Could you check a few things on this model? Use its own coordinates, in mm. A direction names the side the tool comes from. Coordinates: 2 decimals unless noted, no trailing zeros. Write each loop counter-clockwise with the first axis right and the second up, starting at its lowest first coordinate (ties: lowest second). Pieces come first, ordered by that corner, then holes. Notation, with made-up numbers: (0.25, -24.75) - (32.25, -24.75) arc R11 cw to (32.25, -5.75) - close; hole circle Ø1 at (74.25, -17). An arc over 180 degrees is marked (long way). Write item = value, one per line. Start each with the question number.
```python
from build123d import *

# Parameters (mm, degrees)
BOSS_EXTRUDE1_DEPTH = 10
SKETCH2_R           = 7.5
BOSS_EXTRUDE2_DEPTH = 126
CHAMFER1_SIZE       = 1


with BuildPart() as part:
    # Sketch1 → Boss-Extrude1 (new body)
    with BuildSketch(Plane(origin=(0, 0, 0), x_dir=(1, 0, 0), z_dir=(0, 1, 0))):
        Polygon((0, 12.701705922), (-11, 6.350852961), (-11, -6.350852961), (0, -12.701705922), (11, -6.350852961), (11, 6.350852961), align=None)
    extrude(amount=BOSS_EXTRUDE1_DEPTH)

    # Sketch2 → Boss-Extrude2 (add)
    with BuildSketch(Plane.XZ):
        Circle(SKETCH2_R)
    extrude(amount=BOSS_EXTRUDE2_DEPTH)

    # Sketch4 → Cut-Revolve2 (revolve, cut)
    with BuildSketch(Plane(origin=(0, 0, 0), x_dir=(0, 0, -1), z_dir=(1, 0, 0))):
        Polygon((-12.701705922, 10), (-12.701705922, 8.8), (-11.201705922, 10), align=None)
        Polygon((-12.701705922, 0), (-12.701705922, 1.2), (-11.201705922, 0), align=None)
    revolve(axis=Axis((0, 0, 0), (0, 1, 0)), mode=Mode.SUBTRACT)

    # Chamfer1
    chamfer1_edges = [part.edges().sort_by_distance(p)[0] for p in [
        (-7.5, -126, 0),
    ]]
    chamfer(chamfer1_edges, length=CHAMFER1_SIZE)


solid = part.part
```
1) If I drill on probe 1 along Y at (x, z) = (4.5, 6.75); probe 2 along Z at (x, y) = (0.25, -118); probe 3 along Z at (x, y) = (-6.25, -40.5), over which ranges is the centre line in solid material (lowest first)? Write a range as [from, to].
2) For P1, Ø3, axis at x = 7, y = -19, coming from the -Z side; P2, Ø10, axis at x = -6, y = -28, coming from the -Z side; P3, Ø6, axis at x = 3.5, y = -20.5, coming from the -Z side, each with a flat end and sliding along its axis, tell me the tip position at first contact or that it passes through.
3) Suppose I cut it at B-B on y = -89. Please give me the cut outline in (x, z), plus the area to 3 significant figures.
4) Suppose I cut it at A-A on z = 0. Please give me the cut outline in (x, y), plus the area to 3 significant figures.
5) Which directions (+Z, -Z, +X, -X, +Y, -Y) give clear straight access to the entire face, cutting with the end or side of a thin tool? Please do faces 1 (the flat face through (0, 0, -8)), 2 (the conical face through (10.026, 9.675, 5.851)).
Reply:
q1.probe_1 = [0, 10]
q1.probe_2 = [-7.5, 7.5]
q1.probe_3 = [-4.15, 4.15]
q2.P1 = -5.1
q2.P2 = -7.43
q2.P3 = -7.48
q3.outline = circle Ø15 at (0, 0)
q3.area = 177 mm^2
q4.outline = (-11, 0) - (-7.5, 0) - (-7.5, -125) - (-6.5, -126) - (6.5, -126) - (7.5, -125) - (7.5, 0) - (11, 0) - (11, 10) - (-11, 10) - close
q4.area = 2,110 mm^2
q5.face_1 = -Y
q5.face_2 = +Z, +X, +Y
